```python
from build123d import *

# Parameters (mm, degrees)
F0_W     = 168
F0_H     = 68
F0_W_2   = 163
F0_H_2   = 63
F1_DEPTH = 60
F2_DEPTH = 2
F3_W     = 4.826
F3_H     = 24.355216
F4_DEPTH = 3


with BuildPart() as f1:
    # F0 (on Top) → F1 (new body)
    with BuildSketch(Plane.XY):
        Rectangle(F0_W, F0_H)
        Rectangle(F0_W_2, F0_H_2, mode=Mode.SUBTRACT)
    extrude(amount=F1_DEPTH)

    # F0 (on Top) → F2 (join)
    with BuildSketch(Plane.XY):
        Rectangle(F0_W_2, F0_H_2)
    extrude(amount=F2_DEPTH)

    # F3 (on face) → F4 (join)
    with BuildSketch(Plane.XY):
        with BuildLine():
            Line((-60.442161, 24.30206), (-72.00386, 24.30206))
            Line((-72.00386, 24.30206), (-72.208633, 18.363613))
            ThreePointArc((-72.208633, 18.363613), (-71.269145, 14.427374), (-68.446746, 11.527256))
            Line((-68.446746, 11.527256), (-67.12627, 10.753183))
            Line((-67.12627, 10.753183), (-67.12627, 18.882509))
            Line((-67.12627, 18.882509), (-60.442161, 18.882509))
            Line((-60.442161, 18.882509), (-60.442161, 24.30206))
        make_face()
        with BuildLine():
            Line((-47.606919, 24.634736), (-53.000022, 24.634736))
            Line((-53.000022, 24.634736), (-52.930937, -11.566137))
            ThreePointArc((-52.930937, -11.566137), (-51.338734, -16.213165), (-47.241549, -18.922972))
            Line((-47.241549, -18.922972), (-14.994091, -27.368734))
            Line((-14.994091, -27.368734), (-14.994091, -21.587882))
            Line((-14.994091, -21.587882), (-45.218573, -13.409639))
            Line((-45.218573, -13.409639), (-16.646753, 24.478305))
            Line((-16.646753, 24.478305), (-22.944923, 24.478305))
            Line((-22.944923, 24.478305), (-47.740912, -9.533542))
            Line((-47.740912, -9.533542), (-47.606919, 24.634736))
        make_face()
        with BuildLine():
            Line((-5.600203, 16.858305), (-5.600203, -26.761888))
            Line((-5.600203, -26.761888), (-1.264561, -26.761888))
            Line((-1.264561, -26.761888), (-1.264561, 12.522665))
            ThreePointArc((-1.264561, 12.522665), (0.967285, 17.910819), (6.355439, 20.142665))
            Line((6.355439, 20.142665), (28.542969, 20.142665))
            Line((28.542969, 20.142665), (28.542969, 24.478305))
            Line((28.542969, 24.478305), (2.019797, 24.478305))
            ThreePointArc((2.019797, 24.478305), (-3.368357, 22.246459), (-5.600203, 16.858305))
        make_face()
        with BuildLine():
            ThreePointArc((44.653603, 24.478305), (39.265449, 22.246459), (37.033603, 16.858305))
            Line((37.033603, 16.858305), (37.033603, -26.761888))
            Line((37.033603, -26.761888), (42.272501, -26.761888))
            Line((42.272501, -26.761888), (42.272501, 11.980708))
            ThreePointArc((42.272501, 11.980708), (44.504347, 17.368862), (49.892501, 19.600708))
            Line((49.892501, 19.600708), (75.693063, 19.600708))
            Line((75.693063, 19.600708), (75.693063, 24.478305))
            Line((75.693063, 24.478305), (44.653603, 24.478305))
        make_face()
        with Locations((73.283109, -14.58428)):
            Rectangle(F3_W, F3_H)
    extrude(amount=-F4_DEPTH)


solid = f1.part
```
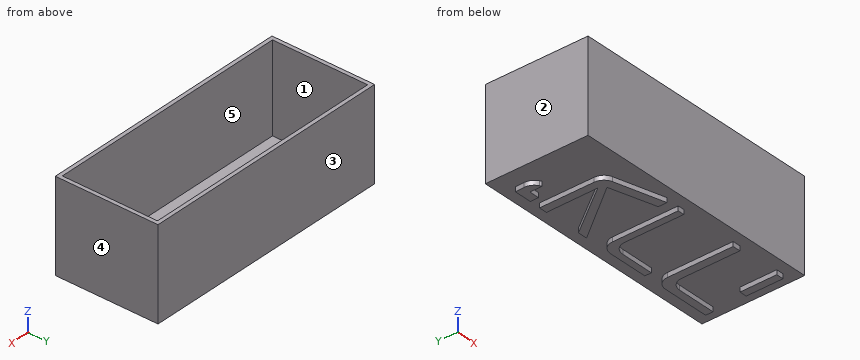
Verification items for the finished model (mm, model axes). Face numbers are marked on the shaded views. A direction names the side the tool comes from. Give positions to 0.01 mm unless a question says otherwise; leave off trailing zeros. Loops run counter-clockwise (first coordinate to the right, second up) from the corner with the lowest first, then second, coordinate; pieces in that order, holes last.
1. Section check D-D, the plane x = 9.5. Enter the section's corners in (y, z).
2. Section check C-C, the plane y = 5. Enter the section's corners in (x, z), then the cut area to 3 significant figures.
3. Section check A-A, the plane z = 40. Enter the section's corners in (x, y).
4. Mould release check, pull along X, two halves, no side actions. Record for the marked faces 3, 4 and 5: released by +X, released by -X, zero draft, split by the parting line, or undercut.
5. Thickness scan on line 1 (Y direction, x = -9, z = 11); line 2 (X direction, y = 19.5, z = 3); line 3 (Z direction, x = 49, y = -10.5). Record the ranges inside material, lowest first.
6. Go/stop test with flat-tipped pins: pin 1 Ø1.5 at (x, z) = (-51.5, -2) entering from +Y; pin 2 Ø2.5 at (y, z) = (-14, -2) entering from -X; pin 3 Ø2.5 at (x, z) = (-3.5, -1.5) entering from -Y. Record where each tip stops, or that it passes through.
7. Set-up check for the marked faces 1 and 2: record each of +Z, -Z, +X, -X, +Y, -Y from which the full face is reachable in a straight line by a thin tool's end or side.
8. Section check B-B, the plane x = -7.5. Enter the section's corners in (y, z), then the cut area to 3 significant figures.
Geometry says:
1. outline: (-34, 0) - (20.14, 0) - (20.14, -3) - (24.48, -3) - (24.48, 0) - (34, 0) - (34, 60) - (31.5, 60) - (31.5, 2) - (-31.5, 2) - (-31.5, 60) - (-34, 60) - close
2. outline: (-84, 0) - (-52.96, 0) - (-52.96, -3) - (-47.68, -3) - (-47.68, 0) - (-37.15, 0) - (-37.15, -3) - (-31.34, -3) - (-31.34, 0) - (-5.6, 0) - (-5.6, -3) - (-1.26, -3) - (-1.26, 0) - (37.03, 0) - (37.03, -3) - (42.27, -3) - (42.27, 0) - (84, 0) - (84, 60) - (81.5, 60) - (81.5, 2) - (-81.5, 2) - (-81.5, 60) - (-84, 60) - close
2. area: 688 mm2
3. outline: (-84, -34) - (84, -34) - (84, 34) - (-84, 34) - close; hole (-81.5, -31.5) - (81.5, -31.5) - (81.5, 31.5) - (-81.5, 31.5) - close
4. face 3: zero draft
4. face 4: released by +X
4. face 5: undercut
5. line 1: y = -34 to -31.5, 31.5 to 34
5. line 2: x = -84 to -81.5, 81.5 to 84
5. line 3: z = 0 to 2
6. pin 1: stops at y = 24.63
6. pin 2: stops at x = -52.84
6. pin 3: stops at y = -26.76
7. face 1: +Z
7. face 2: +Z, -Z, -X, +Y, -Y
8. outline: (-34, 0) - (34, 0) - (34, 60) - (31.5, 60) - (31.5, 2) - (-31.5, 2) - (-31.5, 60) - (-34, 60) - close
8. area: 426 mm2
